```python
from build123d import *

# Parameters (mm, degrees)
F0_W     = 16.8362744153
F0_H     = 2
F1_DEPTH = 20
F0_H_2   = 10
F2_DEPTH = 2


with BuildPart() as f1:
    # F0 (on Top) → F1 (new body)
    with BuildSketch(Plane.XY):
        with BuildLine():
            Line((0, 33), (0, 35))
            ThreePointArc((0, 35), (-24.7487373415, 24.7487373415), (-35, 0))
            Line((-35, 0), (-33, 0))
            ThreePointArc((-33, 0), (-23.3345237792, 23.3345237792), (0, 33))
        make_face()
        with Locations((8.4181372076, 34)):
            Rectangle(F0_W, F0_H)
        with BuildLine():
            Line((-33, 0), (-35, 0))
            ThreePointArc((-35, 0), (-24.7487373415, -24.7487373415), (0, -35))
            Line((0, -35), (0, -33))
            ThreePointArc((0, -33), (-23.3345237792, -23.3345237792), (-33, 0))
        make_face()
        with Locations((8.4181372076, -34)):
            Rectangle(F0_W, F0_H)
    extrude(amount=F1_DEPTH)



with BuildPart() as f1b:
    # F0 (on Top) → F1, piece 2 (new body)
    with BuildSketch(Plane.XY):
        with BuildLine():
            ThreePointArc((-45, 0), (-31.8198051534, 31.8198051534), (0, 45))
            Line((0, 45), (0, 47))
            ThreePointArc((0, 47), (-33.2340187158, 33.2340187158), (-47, 0))
            Line((-47, 0), (-45, 0))
        make_face()
        with Locations((8.4181372076, 46)):
            Rectangle(F0_W, F0_H)
        with BuildLine():
            ThreePointArc((0, -45), (-31.8198051534, -31.8198051534), (-45, 0))
            Line((-45, 0), (-47, 0))
            ThreePointArc((-47, 0), (-33.2340187158, -33.2340187158), (0, -47))
            Line((0, -47), (0, -45))
        make_face()
        with Locations((8.4181372076, -46)):
            Rectangle(F0_W, F0_H)
    extrude(amount=F1_DEPTH)


with BuildPart() as f1_1:
    add(f1.part)

    add(f1b.part)  # F2 merges F1b
    # F0 (on Top) → F2 (join)
    with BuildSketch(Plane.XY):
        with BuildLine():
            ThreePointArc((0, -35), (-24.7487373415, -24.7487373415), (-35, 0))
            Line((-35, 0), (-45, 0))
            ThreePointArc((-45, 0), (-31.8198051534, -31.8198051534), (0, -45))
            Line((0, -45), (0, -35))
        make_face()
        with BuildLine():
            ThreePointArc((-35, 0), (-24.7487373415, 24.7487373415), (0, 35))
            Line((0, 35), (0, 45))
            ThreePointArc((0, 45), (-31.8198051534, 31.8198051534), (-45, 0))
            Line((-45, 0), (-35, 0))
        make_face()
        with Locations((8.4181372076, 40)):
            Rectangle(F0_W, F0_H_2)
        with Locations((8.4181372076, -40)):
            Rectangle(F0_W, F0_H_2)
    extrude(amount=F2_DEPTH)


solid = f1_1.part
```
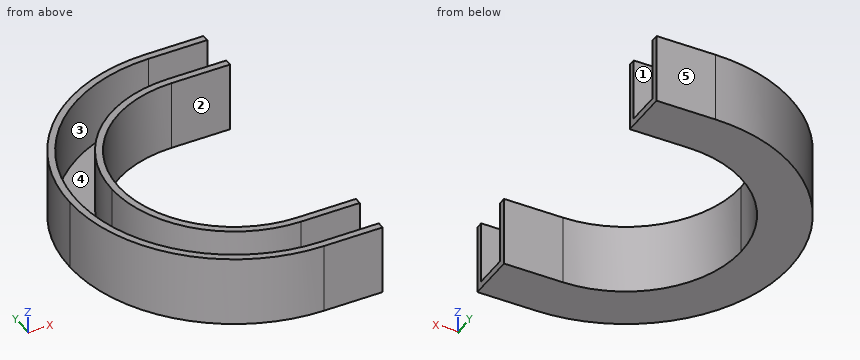
Build history of the part. All positions in model axes, mm. Face numbers are marked on the shaded views. A direction names the side the tool comes from. Give positions to 0.01 mm unless a question says otherwise; leave off trailing zeros. Loops run counter-clockwise (first coordinate to the right, second up) from the corner with the lowest first, then second, coordinate; pieces in that order, holes last.
Item 1: Drill centre lines: line 1 (Y direction, x = 5, z = 4.25); line 2 (Y direction, x = -30, z = 13.25); line 3 (Z direction, x = -17, y = 32.5). Where is each one in solid material? Low to high.
Answers follow:
line 1: y = -47 to -45, -35 to -33, 33 to 35, 45 to 47
line 2: y = -36.18 to -33.54, -18.03 to -13.75, 13.75 to 18.03, 33.54 to 36.18
line 3: z = 0 to 2
Item 2: Pull direction X, two halves, no side cores. Call the marked faces 4 and 5: released by +X, released by -X, zero draft, split by the parting line, or undercut.
Answers follow:
face 4: undercut
face 5: zero draft
Item 3: Flat gauge pins, fed straight in: pin 1 (2 mm diameter, centred on x = -37, z = 15, fed in from +Y); pin 2 (3 mm diameter, centred on y = 13, z = 10, fed in from +X); pin 3 (1.5 mm diameter, centred on y = 28.5, z = 3, fed in from +X); pin 4 (12 mm diameter, centred on x = -10.5, y = -18.5, fed in from -Z). Where does each tip first touch, or does it go through?
Answers follow:
pin 1: stops at y = 30.22
pin 2: stops at x = -29.64
pin 3: stops at x = -15.28
pin 4: passes through
Item 4: Which spindle directions (+Z, -Z, +X, -X, +Y, -Y) get a long thin tool onto all of the face, cutting with end or side? Do the marked faces 1, 2 and 3. Say none if no direction does.
Answers follow:
face 1: +Z, +X
face 2: +Z, -Z, +X
face 3: +Z
Item 5: Slice it at B-B, the plane x = 3.5. List the corners of the cut face in (y, z), and give its area (3 significant figures).
Answers follow:
outline: (-47, 0) - (-33, 0) - (-33, 20) - (-35, 20) - (-35, 2) - (-45, 2) - (-45, 20) - (-47, 20) - close; (33, 0) - (47, 0) - (47, 20) - (45, 20) - (45, 2) - (35, 2) - (35, 20) - (33, 20) - close
area: 200 mm2
Item 6: Slice it at A-A, the plane z = 3.25. List the corners of the cut face in (x, y), and give its area (3 significant figures).
Answers follow:
outline: (0, -47) - (16.84, -47) - (16.84, -45) - (0, -45) arc R45 cw to (0, 45) - (16.84, 45) - (16.84, 47) - (0, 47) arc R47 ccw to start; (0, -35) - (16.84, -35) - (16.84, -33) - (0, -33) arc R33 cw to (0, 33) - (16.84, 33) - (16.84, 35) - (0, 35) arc R35 ccw to start
area: 637 mm2
Item 7: Slice it at D-D, the plane x = -28.5. List the corners of the cut face in (y, z).
Answers follow:
outline: (-37.37, 0) - (-16.64, 0) - (-16.64, 20) - (-20.32, 20) - (-20.32, 2) - (-34.82, 2) - (-34.82, 20) - (-37.37, 20) - close; (16.64, 0) - (37.37, 0) - (37.37, 20) - (34.82, 20) - (34.82, 2) - (20.32, 2) - (20.32, 20) - (16.64, 20) - close
Item 8: Slice it at C-C, the plane y = 37. List the corners of the cut face in (x, z), and give its area (3 significant figures).
Answers follow:
outline: (-28.98, 0) - (16.84, 0) - (16.84, 2) - (-25.61, 2) - (-25.61, 20) - (-28.98, 20) - close
area: 152 mm2
